Verification items for the finished model (mm, model axes). Face numbers are marked on the shaded views. A direction names the side the tool comes from. Coordinates: 2 decimals unless noted, no trailing zeros. Write each loop counter-clockwise with the first axis right and the second up, starting at its lowest first coordinate (ties: lowest second). Pieces come first, ordered by that corner, then holes. Notation, with made-up numbers: (43.25, 51.25) - (76.25, 51.25) arc R22 cw to (76.25, 77.25) - close; hole circle Ø9 at (67, 30). An arc over 180 degrees is marked (long way). Use one line per item in the form item = value. Start each with the question number.
(1) Tool access check on the marked faces 5 and 6. Record the directions out of +Z, -Z, +X, -X, +Y, -Y that give a thin tool (end or side, any length) a straight path to the whole face; none if there is none.
(2) Mould release check, pull along X, two halves, no side actions. Record for the marked faces 1, 2, 3 and 4: released by +X, released by -X, zero draft, split by the parting line, or undercut.
(3) Sectioned sample at B-B (x = 29). Record the cut outline in (y, z).
(4) Gauge pin test, flat end, axial feed: pin 1 Ø2.5 at (x, z) = (37.39, 5) entering from +Y. Record the tip position at first contact, or that the pin passes through.
(5) Sectioned sample at D-D (z = 5). Count the separate pieces of the cut face and the enclosed holes in it, and give its area (3 significant figures).
(6) Sectioned sample at A-A (y = -2). Record the cut outline in (x, z).
(7) Material ranges on line 1 (X direction, y = -11.3, z = 5); line 2 (X direction, y = -7.5, z = 7.5); line 3 (Y direction, x = 6, z = 6), recorded low to high. Write a range as [from, to].
(8) Sectioned sample at C-C (z = 1). Record the cut outline in (x, y), and give its area (3 significant figures).
from build123d import *

# Parameters (mm, degrees)
SKIZZE1_W                                      = 74
SKIZZE1_H                                      = 15
AUFSATZ_LINEAR_AUSTRAGEN1_DEPTH                = 10
SCHNITT_LINEAR_AUSTRAGEN1_REACH                = 61.351
SKIZZE2_W                                      = 71
SKIZZE2_H                                      = 12
FORMSENKUNG_F_R_M3_LINSENSENKSCHRAUB_2_COUNT   = 2
FORMSENKUNG_F_R_M3_LINSENSENKSCHRAUB_2_PITCH   = 34
M3_GEWINDEBOHRUNG1_AT_2_COUNT                  = 2
M3_GEWINDEBOHRUNG1_AT_2_PITCH                  = 65.65
FORMSENKUNG_F_R_M3_LINSENSENKSCHRAUB_3_A_COUNT = 2
FORMSENKUNG_F_R_M3_LINSENSENKSCHRAUB_3_A_PITCH = 49


with BuildPart() as part:
    # Skizze1 → Aufsatz-Linear austragen1 (new body)
    with BuildSketch(Plane.XY):
        with Locations((20.392098069, -3.844827586)):
            Rectangle(SKIZZE1_W, SKIZZE1_H)
    extrude(amount=AUFSATZ_LINEAR_AUSTRAGEN1_DEPTH)

    # Skizze2 → Schnitt-Linear austragen1 (cut, up to next)
    with BuildSketch(Plane.XY.offset(10), mode=Mode.PRIVATE) as schnitt_linear_austragen1_sk1:
        with Locations((20.392098069, -3.844827586)):
            Rectangle(SKIZZE2_W, SKIZZE2_H)
    schnitt_linear_austragen1_tool1 = extrude(schnitt_linear_austragen1_sk1.sketch, amount=-SCHNITT_LINEAR_AUSTRAGEN1_REACH, mode=Mode.PRIVATE) & part.part
    add(schnitt_linear_austragen1_tool1.solids().sort_by_distance((20.392098, -3.844828, 10))[0], mode=Mode.SUBTRACT)

    # Skizze10 → Formsenkung f_r M3 Linsensenkschraube mi (revolve, cut)
    with BuildSketch(Plane(origin=(3.392098069, 3.655172414, 5), x_dir=(0, 0, 1), z_dir=(1, 0, 0))):
        Polygon((0, 0), (0, 1.5), (1.7, 1.5), (1.7, 1.45), (3.15, 0), align=None)
    formsenkung_f_r_m3_linsensenkschraube_mi = revolve(axis=Axis((3.392098069, 10.005172414, 5), (0, -1, 0)), mode=Mode.SUBTRACT)

    # Formsenkung f_r M3 Linsensenkschraub 2: Formsenkung f_r M3 Linsensenkschraube mi ×2
    with Locations(*[(i * FORMSENKUNG_F_R_M3_LINSENSENKSCHRAUB_2_PITCH, 0, 0) for i in range(1, FORMSENKUNG_F_R_M3_LINSENSENKSCHRAUB_2_COUNT)]):
        add(formsenkung_f_r_m3_linsensenkschraube_mi, mode=Mode.SUBTRACT)

    # Skizze12 → M3 Gewindebohrung1 (revolve, cut)
    with BuildSketch(Plane(origin=(53.217098069, 3.655172414, 5), x_dir=(0, 0, 1), z_dir=(1, 0, 0))):
        Polygon((0, 0), (0, 1.5), (1.25, 1.5), (1.25, 0.275), (1.525, 0), align=None)
    m3_gewindebohrung1 = revolve(axis=Axis((53.217098069, 10.005172414, 5), (0, -1, 0)), mode=Mode.SUBTRACT)

    # M3 Gewindebohrung1 at 2: M3 Gewindebohrung1 ×2
    with Locations(*[(-i * M3_GEWINDEBOHRUNG1_AT_2_PITCH, 0, 0) for i in range(1, M3_GEWINDEBOHRUNG1_AT_2_COUNT)]):
        add(m3_gewindebohrung1, mode=Mode.SUBTRACT)

    # Skizze16 → Formsenkung f_r M3 Linsensenkschraub 3 (revolve, cut)
    with BuildSketch(Plane(origin=(44.892098069, -9.844827586, 5), x_dir=(0, 0, 1), z_dir=(1, 0, 0))):
        Polygon((0, 0), (0, 1.5), (1.7, 1.5), (1.7, 1.45), (3.15, 0), align=None)
    formsenkung_f_r_m3_linsensenkschraub_3 = revolve(axis=Axis((44.892098069, -3.494827586, 5), (0, -1, 0)), mode=Mode.SUBTRACT)

    # Formsenkung f_r M3 Linsensenkschraub 3 a: Formsenkung f_r M3 Linsensenkschraub 3 ×2
    with Locations(*[(-i * FORMSENKUNG_F_R_M3_LINSENSENKSCHRAUB_3_A_PITCH, 0, 0) for i in range(1, FORMSENKUNG_F_R_M3_LINSENSENKSCHRAUB_3_A_COUNT)]):
        add(formsenkung_f_r_m3_linsensenkschraub_3, mode=Mode.SUBTRACT)


solid = part.part
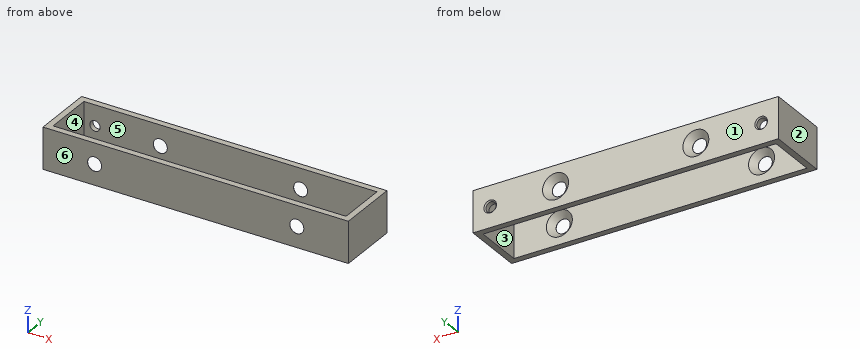
Answers below:
q1.face_5 = +Z, -Z
q1.face_6 = +Z, -Z, +X, -X, -Y
q2.face_1 = zero draft
q2.face_2 = released by -X
q2.face_3 = undercut
q2.face_4 = undercut
q3.outline = (-11.34, 0) - (-9.84, 0) - (-9.84, 10) - (-11.34, 10) - close; (2.16, 0) - (3.66, 0) - (3.66, 10) - (2.16, 10) - close
q4.pin_1 = -9.84
q5.separate_pieces = 6
q5.enclosed_holes = 0
q5.area = 222 mm2
q6.outline = (-16.61, 0) - (-15.11, 0) - (-15.11, 10) - (-16.61, 10) - close; (55.89, 0) - (57.39, 0) - (57.39, 10) - (55.89, 10) - close
q7.line_1 = [-16.61, -5.81], [-2.41, 43.19], [46.59, 57.39]
q7.line_2 = [-16.61, -15.11], [55.89, 57.39]
q7.line_3 = [-11.34, -9.84], [2.16, 3.3]
q8.outline = (-16.61, -11.34) - (57.39, -11.34) - (57.39, 3.66) - (-16.61, 3.66) - close; hole (-15.11, -9.84) - (55.89, -9.84) - (55.89, 2.16) - (-15.11, 2.16) - close
q8.area = 258 mm2
